Here's how the part is built. I have some questions about the finished solid (model axes, mm). A direction names the side the tool comes from. Round coordinates to 2 decimals unless told otherwise and drop trailing zeros. Write each loop counter-clockwise with the first axis right and the second up, starting at its lowest first coordinate (ties: lowest second). Pieces come first, ordered by that corner, then holes. Notation, with made-up numbers: (-30.75, -34) -> (-4.75, -34) arc R25 ccw to (-4.75, -21) -> close; hole circle Ø1 at (29, 73). An arc over 180 degrees is marked (long way). Answer as CSV lines item,"result".
```python
from build123d import *

# Parameters (mm, degrees)
SKETCH1_W           = 30
SKETCH1_H           = 20
SKETCH1_R           = 2.75
BOSS_EXTRUDE1_DEPTH = 5
SKETCH2_W           = 30
SKETCH2_H           = 8
BOSS_EXTRUDE2_DEPTH = 15
SKETCH3_R           = 2.15
CUT_EXTRUDE1_DEPTH  = 6
FILLET1_R           = 1


with BuildPart() as part:
    # Sketch1 → Boss-Extrude1 (new body)
    with BuildSketch(Plane(origin=(0, 0, 0), x_dir=(1, 0, 0), z_dir=(0, 1, 0))):
        with Locations((15, 10)):
            Rectangle(SKETCH1_W, SKETCH1_H)
        with Locations(Location((6.25, 5, 0), (0, 0, 270))):
            Circle(SKETCH1_R, mode=Mode.SUBTRACT)
        with Locations(Location((23.75, 5, 0), (0, 0, 270))):
            Circle(SKETCH1_R, mode=Mode.SUBTRACT)
    extrude(amount=BOSS_EXTRUDE1_DEPTH)

    # Sketch2 → Boss-Extrude2 (add)
    with BuildSketch(Plane(origin=(0, 5, 0), x_dir=(1, 0, 0), z_dir=(0, 1, 0))):
        with Locations((15, 16)):
            Rectangle(SKETCH2_W, SKETCH2_H)
    extrude(amount=BOSS_EXTRUDE2_DEPTH)

    # Sketch3 → Cut-Extrude1 (cut)
    with BuildSketch(Plane(origin=(0, 20, 0), x_dir=(1, 0, 0), z_dir=(0, 1, 0))):
        with Locations(Location((5.25, 16, 0), (0, 0, 270))):
            Circle(SKETCH3_R)
        with Locations(Location((24.75, 16, 0), (0, 0, 270))):
            Circle(SKETCH3_R)
    extrude(amount=-CUT_EXTRUDE1_DEPTH, mode=Mode.SUBTRACT)

    # Fillet1
    fillet1_edges = [part.edges().sort_by_distance(p)[0] for p in [
        (30, 5, -6),
        (0, 5, -6),
        (15, 5, -12),
        (0, 12.5, -12),
        (30, 12.5, -12),
        (0, 20, -16),
        (15, 20, -12),
        (30, 20, -16),
        (15, 20, -20),
        (15, 0, -20),
        (30, 0, -10),
        (15, 0, 0),
        (0, 0, -10),
        (0, 10, -20),
        (30, 10, -20),
        (30, 2.5, 0),
        (0, 2.5, 0),
        (15, 5, 0),
    ]]
    fillet(fillet1_edges, radius=FILLET1_R)


solid = part.part
```
1. If I drill on line 1 (X direction, y = 2.2, z = -5); line 2 (X direction, y = 15.55, z = -16); line 3 (Y direction, x = 23.75, z = -15.5), over which ranges is the centre line in solid material (lowest first)?
Numbers:
line 1,"x = 0 to 3.5, 9 to 21, 26.5 to 30"
line 2,"x = 0 to 3.1, 7.4 to 22.6, 26.9 to 30"
line 3,"y = 0 to 14"
2. Suppose I cut it at A-A on z = -5. Please give me the cut outline in (x, y).
Numbers:
outline,"(0, 1) arc R1 ccw to (1, 0) -> (3.5, 0) -> (3.5, 5) -> (1, 5) arc R1 ccw to (0, 4) -> close; (9, 0) -> (21, 0) -> (21, 5) -> (9, 5) -> close; (26.5, 0) -> (29, 0) arc R1 ccw to (30, 1) -> (30, 4) arc R1 ccw to (29, 5) -> (26.5, 5) -> close"
3. For pin 1 Ø9 at (x, z) = (6.25, -5) entering from +Y; pin 2 Ø5 at (x, y) = (16, 16) entering from +Z; pin 3 Ø2 at (x, z) = (24.5, -16.5) entering from +Y; pin 4 Ø3.5 at (x, z) = (23.75, -5) entering from +Y, each with a flat end and sliding along its axis, tell me the tip position at first contact or that it passes through.
Numbers:
pin 1,"stops at y = 5"
pin 2,"stops at z = -12"
pin 3,"stops at y = 14"
pin 4,"passes through"
4. Suppose I cut it at D-D on z = -16. Please give me the cut outline in (x, y).
Numbers:
outline,"(0, 1) arc R1 ccw to (1, 0) -> (29, 0) arc R1 ccw to (30, 1) -> (30, 19) arc R1 ccw to (29, 20) -> (26.9, 20) -> (26.9, 14) -> (22.6, 14) -> (22.6, 20) -> (7.4, 20) -> (7.4, 14) -> (3.1, 14) -> (3.1, 20) -> (1, 20) arc R1 ccw to (0, 19) -> close"
5. On a 3-axis mill with a long thin cutter (end or side, diameter ignored), from which of +Z, -Z, +X, -X, +Y, -Y can I reach the whole of each face in a straight line? I mean faces 5 (the face through (29.699, 12.591, -12.285)), 6 (the face through (0.285, 12.591, -12.301)), 7 (the face through (15, 5, -6)), 8 (the face through (29.699, 19.715, -16.042)), 9 (the face through (15.196, 0.285, -0.301)). Say none if no direction works.
Numbers:
face 5,"+Z, +X, +Y"
face 6,"+Z, -X, +Y"
face 7,"+Z, +X, -X, +Y"
face 8,"+Z, -Z, +X, +Y"
face 9,"+Z, +X, -X, -Y"
6. If we mould it in two halves opening along Z, with no side actions, what happens to faces 1 (the face through (26.477, 2.465, -5.358)), 2 (the face through (15.196, 4.699, -0.285)), 3 (the face through (5, 14, -16)), 4 (the face through (29.699, 9.874, -19.715))? For each: released by +Z, released by -Z, zero draft, split by the parting line, or undercut.
Numbers:
face 1,"undercut"
face 2,"released by +Z"
face 3,"undercut"
face 4,"released by -Z"
7. Suppose I cut it at C-C on x = 24.75. Please give me the cut outline in (y, z).
Numbers:
outline,"(0, -19) arc R1 ccw to (1, -20) -> (19, -20) arc R1 ccw to (20, -19) -> (20, -18.15) -> (14, -18.15) -> (14, -13.85) -> (20, -13.85) -> (20, -13) arc R1 ccw to (19, -12) -> (6, -12) arc R1 cw to (5, -11) -> (5, -7.56) -> (0, -7.56) -> close; (0, -2.44) -> (5, -2.44) -> (5, -1) arc R1 ccw to (4, 0) -> (1, 0) arc R1 ccw to (0, -1) -> close"
8. Suppose I cut it at B-B on y = 2.75. Please give me the cut outline in (x, z), and give its area (3 significant figures).
Numbers:
outline,"(0, -19) arc R1 ccw to (1, -20) -> (29, -20) arc R1 ccw to (30, -19) -> (30, -1) arc R1 ccw to (29, 0) -> (1, 0) arc R1 ccw to (0, -1) -> close; hole circle Ø5.5 at (6.25, -5); hole circle Ø5.5 at (23.75, -5)"
area,"552 mm^2"
